Autodesk Inventor part; units mm, degrees
ref_plane "YZ Plane" through (0, 0, 0) normal (1, 0, 0) x (0, 1, 0)
ref_plane "XZ Plane" through (0, 0, 0) normal (0, 1, 0) x (-1, 0, 0)
ref_plane "XY Plane" through (0, 0, 0) normal (0, 0, 1) x (1, 0, 0)
sketch "Skizze1" plane through (0, 0, 0) normal (0, 1, 0) x (-1, 0, 0)
  line L0 (-50, 27) -> (50, 27)
  line L1 (50, 27) -> (50, -27) construction
  line L2 (50, -27) -> (-50, -27)
  line L3 (-50, -27) -> (-50, 27)
  line L4 (-50, 27) -> (50, -27) construction
  line L5 (50, 27) -> (-50, -27) construction
  line L6 (0, 0) -> (66.4326, 0) construction
  arc A0 (18, -27) -> (18, 27) centre (18, 0) ccw
  dimension "d0" = 54
  dimension "d1" = 100
  dimension "d12" = 68
  dimension "d13" = 90
extrude "Extrusion1" add sketch "Skizze1" along normal blind 4
sketch "Skizze5" plane through (0, 4, 0) normal (0, 1, 0) x (1, 0, 0)
  line L0 (-18, -27) -> (50, -27)
  line L1 (50, -27) -> (50, 27)
  line L2 (50, 27) -> (-18, 27)
  arc A0 (-18, 27) -> (-18, -27) centre (-18, 0) ccw
  line L3 (35, -27) -> (30, -27)
  line L4 (30, -27) -> (30, 27)
  line L5 (30, 27) -> (35, 27)
  line L6 (35, 27) -> (35, -27)
  point P0 (0, 0)
  dimension "d14" = 15
  dimension "d15" = 5
extrude "Extrusion4" add sketch "Skizze5" along normal blind 5 contours L4 L2 L6 L0
sketch "Skizze6" plane through (0, 4, 0) normal (0, 1, 0) x (1, 0, 0)
  line L0 (35, 27) -> (35, -27)
  line L1 (35, -27) -> (50, -27)
  line L2 (50, -27) -> (50, 27)
  line L3 (50, 27) -> (35, 27)
  line L4 (0, 0) -> (67.4565, 0) construction
  point P0 (46.5, 0)
  dimension "d18" = 3.5
hole "Bohrung1" at (46.5, 4, 0) direction (0, -1, 0) diameter 3.4 end through all
pattern_linear "Rechteckige Anordnung1" count 5 spacing 11 along (0, 0, -1) count 2 spacing 8 along (-1, 0, 0) of "Bohrung1" first direction both ways yes
sketch "Skizze7" plane through (0, 0, 0) normal (0, -1, 0) x (1, 0, 0)
  arc A0 (-18, 27) -> (-18, -27) centre (-18, 0) ccw
  line L0 (-6, 12) -> (-30, 12)
  line L1 (-30, 12) -> (-30, -12)
  line L2 (-30, -12) -> (-6, -12)
  line L3 (-6, -12) -> (-6, 12)
  line L4 (-6, 12) -> (-30, -12) construction
  line L5 (-36, 18) -> (0, -18) construction
  circle A1 centre (-18, 0) radius 18
  line L6 (-18, 22.4057) -> (-18, -22.4722) construction
  line L7 (3.1609, 0) -> (-39.488, 0) construction
  point P0 (0, 0)
  point P1 (-18, -18)
  point P2 (-36, 0)
  point P3 (-18, 18)
  point P4 (0, 0)
  dimension "d32" = 24
  dimension "d33" = 24
  dimension "d35" = 36
hole "Bohrung2" at (-18, 0, -18) at (-36, 0, 0) at (-18, 0, 18) at (0, 0, 0) at (-6, 0, -12) at (-30, 0, -12) at (-30, 0, 12) at (-6, 0, 12) direction (0, 1, 0) diameter 3.4 end through all
properties part number "dynamixel_pro_frame_part3" material "Aluminium 6061"
Can you work these out from the model? Positions are in its coordinate system, mm. A direction names the side the tool comes from. Coordinates: 2 decimals unless noted, no trailing zeros. Write each loop counter-clockwise with the first axis right and the second up, starting at its lowest first coordinate (ties: lowest second). Pieces come first, ordered by that corner, then holes. Notation, with made-up numbers: (52, 57) - (65, 57) arc R20 ccw to (65, 81) - close; hole circle Ø1 at (18, -18.75). An arc over 180 degrees is marked (long way). Return JSON: item names as keys, results as strings. Group by question number.
Item 1: If we section it at B-B (y = 1.25): Count the separate pieces of the cut face and the enclosed holes in it, then the cut area to 3 significant figures.
Item 2: We'd pull the mould along X, two halves only. Please class faces 1 (the face through (-17.35, 2.03, -19.57)), 2 (the face through (50, 2, 0)), 3 (the face through (30, 6, 0)): pulls with the +X half, pulls with the -X half, needs draft (parallel to the pull), parting line crosses it, or undercut.
Item 3: If we section it at C-C (z = 22): Write out the boundary of the cut face in (x, y).
Item 4: If we section it at A-A (x = 46.5): Write out the boundary of the cut face in (y, z).
Item 5: Please list where these lines run through material, in increasing order: probe 1 along Z at (x, y) = (46.5, 1.5); probe 2 along Z at (x, y) = (-30, 1.35); probe 3 along Y at (x, z) = (-14, 13).
Item 6: Which directions (+Z, -Z, +X, -X, +Y, -Y) give clear straight access to the entire face, cutting with the end or side of a thin tool? Please do faces 4 (the face through (-34.34, 2.03, 0.37)), 5 (the face through (-7, 4, 0)), 6 (the face through (35, 6, 0)).
Item 7: If we section it at D-D (x = 0): Write out the boundary of the cut face in (y, z), then the cut area to 3 significant figures.
Item 8: I'm going to push flat-ended pins straight in: pin 1 Ø8 at (x, z) = (15, -13) entering from +Y; pin 2 Ø5 at (y, z) = (1.5, 10.5) entering from -X; pin 3 Ø4 at (y, z) = (7, -15.5) entering from +X. Where does each tip first touch, or does it pass through?
Return value:
{
 "1": {"separate pieces": "1", "enclosed holes": "18", "area": "4,650 mm^2"},
 "2": {"face 1": "undercut", "face 2": "pulls with the +X half", "face 3": "pulls with the -X half"},
 "3": {"outline": "(-33.65, 0) - (36.8, 0) - (36.8, 4) - (35, 4) - (35, 9) - (30, 9) - (30, 4) - (-33.65, 4) - close; (40.2, 0) - (44.8, 0) - (44.8, 4) - (40.2, 4) - close; (48.2, 0) - (50, 0) - (50, 4) - (48.2, 4) - close"},
 "4": {"outline": "(0, -27) - (4, -27) - (4, -23.7) - (0, -23.7) - close; (0, -20.3) - (4, -20.3) - (4, -12.7) - (0, -12.7) - close; (0, -9.3) - (4, -9.3) - (4, -1.7) - (0, -1.7) - close; (0, 1.7) - (4, 1.7) - (4, 9.3) - (0, 9.3) - close; (0, 12.7) - (4, 12.7) - (4, 20.3) - (0, 20.3) - close; (0, 23.7) - (4, 23.7) - (4, 27) - (0, 27) - close"},
 "5": {"probe 1": "z = -27 to -23.7, -20.3 to -12.7, -9.3 to -1.7, 1.7 to 9.3, 12.7 to 20.3, 23.7 to 27", "probe 2": "z = -24.19 to -13.7, -10.3 to 10.3, 13.7 to 24.19", "probe 3": "y = 0 to 4"},
 "6": {"face 4": "+Y, -Y", "face 5": "+Z, -Z, -X, +Y", "face 6": "+Z, -Z, +X, +Y"},
 "7": {"outline": "(0, -27) - (4, -27) - (4, -1.7) - (0, -1.7) - close; (0, 1.7) - (4, 1.7) - (4, 27) - (0, 27) - close", "area": "202 mm^2"},
 "8": {"pin 1": "stops at y = 4", "pin 2": "stops at x = -43.79", "pin 3": "stops at x = 35"}
}
